```python
from build123d import *

# Parameters (mm, degrees)
SKETCH_1_R          = 4.5
EXTRUDE_1_DEPTH     = 8
SKETCH_5_R          = 8
CUT_EXTRUDE_2_DEPTH = 1.5
EXTRUDE_3_REACH     = 74.919
SKETCH_4_R          = 19
SKETCH_4_3_R        = 17.5
CUT_EXTRUDE_3_DEPTH = 73.918862941


with BuildPart() as part:
    # 草圖1 → 填料-伸長1 (new body)
    with BuildSketch(Plane(origin=(0, 0, 0), x_dir=(1, 0, 0), z_dir=(0, 1, 0))):
        with BuildLine():
            ThreePointArc((-40.134328358, -5.816588533), (-42, 0), (-40.134328358, 5.816588533))
            ThreePointArc((-40.134328358, 5.816588533), (-16, 27.712812921), (15.029850746, 37.665642188))
            ThreePointArc((15.029850746, 37.665642188), (21, 36.373066959), (25.104477612, 31.849053656))
            ThreePointArc((25.104477612, 31.849053656), (32, 0), (25.104477612, -31.849053656))
            ThreePointArc((25.104477612, -31.849053656), (21, -36.373066959), (15.029850746, -37.665642188))
            ThreePointArc((15.029850746, -37.665642188), (-16, -27.712812921), (-40.134328358, -5.816588533))
        make_face()
        with Locations((-32, 0)):
            Circle(SKETCH_1_R, mode=Mode.SUBTRACT)
        with Locations((16, 27.712812921)):
            Circle(SKETCH_1_R, mode=Mode.SUBTRACT)
        with Locations((16, -27.712812921)):
            Circle(SKETCH_1_R, mode=Mode.SUBTRACT)
    extrude(amount=EXTRUDE_1_DEPTH)

    # 草圖5 → 除料-伸長2 (cut)
    with BuildSketch(Plane(origin=(0, 8, 0), x_dir=(1, 0, 0), z_dir=(0, 1, 0))):
        with Locations((-32, 0)):
            Circle(SKETCH_5_R)
        with Locations((16, 27.712812921)):
            Circle(SKETCH_5_R)
        with Locations((16, -27.712812921)):
            Circle(SKETCH_5_R)
    extrude(amount=-CUT_EXTRUDE_2_DEPTH, mode=Mode.SUBTRACT)

    # 填料-伸長3: up to this face of the body (flat: up to its plane)
    extrude_3_end = Plane(part.part.faces().sort_by_distance((0, 8, 0))[0])
    # 草圖4 → 填料-伸長3 (add, up to the picked face)
    with BuildSketch(Plane(origin=(23.315382908, 50, 0), x_dir=(0.906307787, -0.422618262, 0), z_dir=(0.422618262, 0.906307787, 0)), mode=Mode.PRIVATE) as extrude_3_sk1:
        Circle(SKETCH_4_R)
    extrude_3_tool1 = split(extrude(extrude_3_sk1.sketch, amount=-EXTRUDE_3_REACH, mode=Mode.PRIVATE), bisect_by=extrude_3_end, keep=Keep.BOTH, mode=Mode.PRIVATE)
    add(extrude_3_tool1.solids().sort_by_distance((23.315383, 50, 0))[0])

    # 草圖4<3> → 除料-伸長3 (cut, through all)
    with BuildSketch(Plane(origin=(23.315382908, 50, 0), x_dir=(0.906307787, -0.422618262, 0), z_dir=(0.422618262, 0.906307787, 0))):
        Circle(SKETCH_4_3_R)
    extrude(amount=-CUT_EXTRUDE_3_DEPTH, mode=Mode.SUBTRACT)


solid = part.part
```
Geometry check sheet. Reference: the model listing, model coordinates, mm. A direction names the side the tool comes from. Give positions to 0.01 mm unless a question says otherwise; leave off trailing zeros. Loops run counter-clockwise (first coordinate to the right, second up) from the corner with the lowest first, then second, coordinate; pieces in that order, holes last. Notation, with made-up numbers: M -23.5,57 L -10.5,57 A21 ccw -10.5,86 Z; hole C 76.5,-10.75 d1. An arc over 180 degrees is marked long. Write item = value, one per line. Start each with the question number.
1. Go/stop test with flat-tipped pins: P1, Ø8, axis at x = -30.5, z = -0.5, coming from the +Y side; P2, Ø4, axis at y = 39, z = -18.5, coming from the +X side; P3, Ø2, axis at y = 35.5, z = 18, coming from the +X side. Record where each tip stops, or that it passes through.
2. Section check C-C, the plane x = -21. Enter the section's corners in (y, z), plus the area to 3 significant figures.
3. Section check B-B, the plane z = 0. Enter the section's corners in (x, y) (3 decimals), plus the area to 3 significant figures.
4. Tool access check on faces 1 (the face through (9.651, 7.26, -22.845)), 2 (the face through (12.43, 3.2, -24.97)), 3 (the face through (-42, 4, 0)), 4 (the face through (-21, 8, -1)), 5 (the face through (32, 4, 0)). Record the directions out of +Z, -Z, +X, -X, +Y, -Y that give a thin tool (end or side, any length) a straight path to the whole face; none if there is none.
5. Section check A-A, the plane x = -30. Enter the section's corners in (y, z).
6. Thickness scan on probe 1 along Z at (x, y) = (-3, 30.5); probe 2 along Y at (x, z) = (26, 0); probe 3 along Z at (x, y) = (29.5, 44). Record the ranges inside material, lowest first.
7. Draft check along X on faces 6 (the face through (38.54, 42.9, 5.54)), 7 (the face through (9.65, 7.26, 32.58)), 8 (the face through (-16.4, 3.94, -27.48)). Enter one of: +X half, -X half, draft (parallel to the pull), parting line (faces both ways), or undercut.
Values follow:
q1.P1 = 6.5
q1.P2 = 28.69
q1.P3 = 25.96
q2.outline = M 0,-24.56 L 8,-24.56 L 8,24.56 L 0,24.56 Z
q2.area = 393 mm^2
q3.outline = M -42,0 L -36.5,0 L -36.5,6.5 L -40,6.5 L -40,8 L -42,8 Z; M -27.5,0 L -19.309,0 L 7.455,57.396 L 6.096,58.03 L -17.234,8 L -24,8 L -24,6.5 L -27.5,6.5 Z; M 19.309,0 L 32,0 L 32,8 L 24.695,8 L 40.535,41.97 L 39.176,42.604 Z
q3.area = 340 mm^2
q4.face_1 = +Y
q4.face_2 = +Y, -Y
q4.face_3 = -X, +Y, -Y
q4.face_4 = none
q4.face_5 = +X, -Y
q5.outline = M 0,-17.36 L 8,-17.36 L 8,-7.75 L 6.5,-7.75 L 6.5,-4.03 L 0,-4.03 Z; M 0,4.03 L 6.5,4.03 L 6.5,7.75 L 8,7.75 L 8,17.36 L 0,17.36 Z
q6.probe_1 = -10.83 to -7.91, 7.91 to 10.83
q6.probe_2 = 0 to 8, 10.8 to 14.35
q6.probe_3 = -17.17 to -15.49, 15.49 to 17.17
q7.face_6 = +X half
q7.face_7 = undercut
q7.face_8 = -X half
